Build history of the part. All positions in model axes, mm. A direction names the side the tool comes from. Give positions to 0.01 mm unless a question says otherwise; leave off trailing zeros. Write each loop counter-clockwise with the first axis right and the second up, starting at its lowest first coordinate (ties: lowest second). Pieces come first, ordered by that corner, then holes. Notation, with made-up numbers: (38, 38.5) -> (67, 38.5) arc R28 cw to (67, 57.5) -> close; hole circle Ø8 at (53, 24). An arc over 180 degrees is marked (long way). Put each result on its own line as item: value. Start each with the question number.
Item 1: Slice it at A-A, the plane z = 0.65. List the corners of the cut face in (x, y), plus the area to 3 significant figures.
Item 2: Slice it at B-B, the plane y = -16.5. List the corners of the cut face in (x, z).
Item 3: Two-plate mould, pull along X, no slides. Class faces 1 (the flat face through (8.6, 0.3, 0)), 2 (the cylindrical face through (12.587, -12.867, 0.986)), 3 (the cylindrical face through (-4.336, -19.524, 0.986)): pulls with the +X half, pulls with the -X half, needs draft (parallel to the pull), parting line crosses it, or undercut.
Item 4: Tool access for faces 4 (the flat face through (0, -7.3, 3)), 5 (the flat face through (-5, -9, 2)), 6 (the flat face through (0, 13, 1)): list every direction of +Z, -Z, +X, -X, +Y, -Y with a clear straight run to the whole face (end or side of a thin tool).
Item 5: Drill centre lines: line 1 along Y through (x, z) = (-5.5, 1.5); line 2 along Y through (x, z) = (6, 0.5); line 3 along Y through (x, z) = (0, 2.15). Where is each one in solid material? Low to high.
Item 6: Slice it at C-C, the plane x = -14.5. List the corners of the cut face in (y, z).
Item 7: Flat gauge pins, fed straight in: pin 1 Ø1.6 at (x, z) = (13.5, 1.5) entering from -Y; pin 2 Ø1.5 at (x, z) = (7, 2.5) entering from +Y; pin 3 Ø1.6 at (y, z) = (-11.5, 1.5) entering from +X. Where does each tip first touch, or does it go through?
Item 8: Slice it at D-D, the plane y = 4.5. List the corners of the cut face in (x, z), plus the area to 3 significant figures.
```python
from build123d import *

# Parameters (mm, degrees)
TUBE002_R     = 9
TUBE002_R_2   = 7
TUBE002_DEPTH = 3
BOX001_W      = 20
BOX001_H      = 20
BOX001_DEPTH  = 10
BOX_W         = 20
BOX_H         = 20
BOX_DEPTH     = 10
TUBE_R        = 18
TUBE_R_2      = 9
TUBE_DEPTH    = 10
TUBE001_R     = 20
TUBE001_R_2   = 7
TUBE001_DEPTH = 2


with BuildPart() as tube002:
    # Tube002 → Tube002 (new body)
    with BuildSketch(Plane.XY):
        Circle(TUBE002_R)
        Circle(TUBE002_R_2, mode=Mode.SUBTRACT)
    extrude(amount=TUBE002_DEPTH)


with BuildPart() as cubo001:
    # Box001 → Box001 (new body)
    with BuildSketch(Plane(origin=(-20, -20, 0), x_dir=(1, 0, 0), z_dir=(0, 0, 1))):
        with Locations((10, 10)):
            Rectangle(BOX001_W, BOX001_H)
    extrude(amount=BOX001_DEPTH)


with BuildPart() as cubo:
    # Box → Box (new body)
    with BuildSketch(Plane.XY):
        with Locations((10, 10)):
            Rectangle(BOX_W, BOX_H)
    extrude(amount=BOX_DEPTH)


with BuildPart() as cut001:
    # Tube → Tube (new body)
    with BuildSketch(Plane.XY):
        Circle(TUBE_R)
        Circle(TUBE_R_2, mode=Mode.SUBTRACT)
    extrude(amount=TUBE_DEPTH)

    # Cut: cut Cubo
    add(cubo.part, mode=Mode.SUBTRACT)

    # Cut001: cut Cubo001
    add(cubo001.part, mode=Mode.SUBTRACT)


with BuildPart() as fusion:
    # Tube001 → Tube001 (new body)
    with BuildSketch(Plane.XY):
        Circle(TUBE001_R)
        Circle(TUBE001_R_2, mode=Mode.SUBTRACT)
    extrude(amount=TUBE001_DEPTH)

    # Cut002: cut Cut001
    add(cut001.part, mode=Mode.SUBTRACT)

    # Fusion: union Tube002
    add(tube002.part)


solid = fusion.part
```
Values follow:
1. outline: circle Ø40 at (0, 0); hole (-18, 0) -> (-9, 0) arc R9 cw to (0, 9) -> (0, 18) arc R18 ccw to start; hole circle Ø14 at (0, 0); hole (0, -18) arc R18 ccw to (18, 0) -> (9, 0) arc R9 cw to (0, -9) -> close
1. area: 721 mm2
2. outline: (-11.3, 0) -> (0, 0) -> (0, 2) -> (-11.3, 2) -> close; (7.19, 0) -> (11.3, 0) -> (11.3, 2) -> (7.19, 2) -> close
3. face 1: needs draft
3. face 2: undercut
3. face 3: parting line crosses it
4. face 4: +Z, +X, -X, +Y, -Y
4. face 5: +Z
4. face 6: +Z, -Z
5. line 1: -19.23 to -4.33, 4.33 to 7.12, 17.14 to 19.23
5. line 2: -19.08 to -16.97, -6.71 to -3.61, 3.61 to 19.08
5. line 3: -9 to -7, 7 to 9
6. outline: (-13.77, 0) -> (0, 0) -> (0, 2) -> (-13.77, 2) -> close; (10.67, 0) -> (13.77, 0) -> (13.77, 2) -> (10.67, 2) -> close
7. pin 1: y = -15.45
7. pin 2: y = 18.93
7. pin 3: x = 16.9
8. outline: (-19.49, 0) -> (-17.43, 0) -> (-17.43, 2) -> (-19.49, 2) -> close; (-7.79, 0) -> (-5.36, 0) -> (-5.36, 3) -> (-7.79, 3) -> close; (5.36, 0) -> (19.49, 0) -> (19.49, 2) -> (7.79, 2) -> (7.79, 3) -> (5.36, 3) -> close
8. area: 42.1 mm2
